Source: CAD feature listing. Evaluate the final solid. Frame: model axes, mm. Give positions to 0.01 mm unless a question says otherwise; leave off trailing zeros. Loops run counter-clockwise (first coordinate to the right, second up) from the corner with the lowest first, then second, coordinate; pieces in that order, holes last. Notation, with made-up numbers: M 84.5,-12 L 111.5,-12 A29 cw 111.5,23 Z; hole C -3.75,-12 d8. An arc over 180 degrees is marked long. Put each result on its own line as item: value. Start each with the question number.
```python
from build123d import *

# Parameters (mm, degrees)
SKETCH1_R           = 14.1
SKETCH1_R_2         = 6
BOSS_EXTRUDE1_DEPTH = 8.1
FILLET1_R           = 0.5


with BuildPart() as part:
    # Sketch1 → Boss-Extrude1 (new body)
    with BuildSketch(Plane.XY):
        with Locations(Location((1.959493634, 6.335e-06, 0), (0, 0, 270))):
            Circle(SKETCH1_R)
        with Locations(Location((1.959493634, 6.335e-06, 0), (0, 0, 270))):
            Circle(SKETCH1_R_2, mode=Mode.SUBTRACT)
    extrude(amount=BOSS_EXTRUDE1_DEPTH)

    # Fillet1
    fillet1_edges = [part.edges().sort_by_distance(p)[0] for p in [
        (1.959493634, 14.100006335, 8.1),
        (1.959493634, 14.100006335, 0),
        (1.959493634, 6.000006335, 0),
        (1.959493634, 6.000006335, 8.1),
    ]]
    fillet(fillet1_edges, radius=FILLET1_R)


solid = part.part
```
1. Section A-A, the plane z = 4.5. Output: boundary loops of the cut face in (x, y).
2. Contact query for flat-ended pins moving along their axis: pin 1 (12 mm diameter, centred on x = 1, y = 5.5, fed in from -Z); pin 2 (3 mm diameter, centred on y = 9.5, z = 5, fed in from -X); pin 3 (3 mm diameter, centred on y = 2, z = 5, fed in from -X); pin 4 (1.5 mm diameter, centred on x = 9.5, z = 4.5, fed in from -Y). Output: stop coordinate, or through.
3. Ray query, line 1 (X direction, y = -2.5, z = 6.75); line 2 (Y direction, x = 7, z = 7.25); line 3 (X direction, y = 4.75, z = 6.5). Return the intervals inside material, ascending.
4. Pull-direction query (Y, two-part tool) for faces 1 (the face through (13.85, -7.58, 4)), 2 (the face through (7.91, 0.78, 4)), 3 (the face through (-1, -6, 0)); classes: released by +Y, released by -Y, zero draft, split by the parting line, or undercut.
Results found:
1. outline: C 1.96,0 d28.2; hole C 1.96,0 d12
2. pin 1: z = 0
2. pin 2: x = -9.65
2. pin 3: x = -12.13
2. pin 4: y = -12.36
3. line 1: -11.92 to -3.49, 7.41 to 15.84
3. line 2: -13.17 to -3.25, 3.25 to 13.17
3. line 3: -11.32 to -1.71, 5.63 to 15.24
4. face 1: split by the parting line
4. face 2: undercut
4. face 3: zero draft
